```python
from build123d import *

# Parameters (mm, degrees)
BOSS_EXTRUDE1_DEPTH = 55
SKETCH2_W           = 14.545162339
SKETCH2_H           = 14.545162338
CUT_EXTRUDE1_DEPTH  = 55
SKETCH3_W           = 7.673243051
SKETCH3_H           = 2.777107306
SKETCH3_W_2         = 8.184792588
CUT_EXTRUDE2_DEPTH  = 55
SKETCH4_R           = 2.665972182
CUT_EXTRUDE3_DEPTH  = 20
FILLET1_R           = 12.5


with BuildPart() as part:
    # Sketch1 → Boss-Extrude1 (new body)
    with BuildSketch(Plane.XY):
        Polygon((41.400095641, 5), (28.900095641, 5), (-2.499905164, 5), (-2.499905164, 10), (-22.499903554, 10), (-22.499903554, 5), (-28.900095641, 5), (-41.400095641, 5), (-41.400095641, -10), (-28.900095641, -10), (28.900095641, -10), (41.400095641, -10), align=None)
    extrude(amount=BOSS_EXTRUDE1_DEPTH)

    # Sketch2 → Cut-Extrude1 (cut)
    with BuildSketch(Plane(origin=(0, 5, 0), x_dir=(1, 0, 0), z_dir=(0, 1, 0))):
        with Locations((23.65160359, -27.5)):
            Rectangle(SKETCH2_W, SKETCH2_H)
    extrude(amount=-CUT_EXTRUDE1_DEPTH, mode=Mode.SUBTRACT)

    # Sketch3 → Cut-Extrude2 (cut)
    with BuildSketch(Plane(origin=(-2.499905164, 0, 0), x_dir=(0, 0, -1), z_dir=(1, 0, 0))):
        with Locations((-47.272594324, 6.388553653)):
            Rectangle(SKETCH3_W, SKETCH3_H)
        with Locations((-8.522716918, 6.388553653)):
            Rectangle(SKETCH3_W_2, SKETCH3_H)
    extrude(amount=-CUT_EXTRUDE2_DEPTH, mode=Mode.SUBTRACT)

    # Sketch4 → Cut-Extrude3 (cut)
    with BuildSketch(Plane(origin=(41.400095641, 0, 0), x_dir=(0, 0, -1), z_dir=(1, 0, 0))):
        with Locations((-27.5, -2.516392759)):
            Circle(SKETCH4_R)
    extrude(amount=-CUT_EXTRUDE3_DEPTH, mode=Mode.SUBTRACT)

    # Fillet1
    fillet1_edges = [part.edges().sort_by_distance(p)[0] for p in [
        (-41.400095641, -2.5, 0),
        (41.400095641, -2.5, 0),
        (-41.400095641, -2.5, 55),
        (41.400095641, -2.5, 55),
    ]]
    fillet(fillet1_edges, radius=FILLET1_R)


solid = part.part
```
Work out the finished part from the listing and answer in its coordinate system (mm). A direction names the side the tool comes from. Give positions to 0.01 mm unless a question says otherwise; leave off trailing zeros. Order: outer loops, then holes, each group sorted by start corner. A loop starts at its lowest first (then second) coordinate and runs counter-clockwise, first axis right, second up. Notation, with made-up numbers: (62, 7.25) -> (81, 7.25) arc R23 cw to (81, 39.25) -> close; hole circle Ø10 at (-14.75, 79). An arc over 180 degrees is marked (long way). Answer as CSV lines item,"result". Start each with the question number.
(1) Consider line 1 along X through (y, z) = (-1, 21); line 2 along Y through (x, z) = (33.5, 27.5); line 3 along X through (y, z) = (8, 30). Determine where each line is inside the solid, lowest interval first.
(2) For a pull along X with two mould halves and no side action, classify faces 5 (the flat face through (-12, 7.777, 9)), 6 (the cylindrical face through (37.836, -2.395, 51.241)), 7 (the flat face through (-22.5, 8, 27)), 8 (the flat face through (24, -2, 20.227)) as released by +X, released by -X, zero draft, split by the parting line, or undercut.
(3) Section C-C, the plane x = -20.5 is taken. Write down the section's boundary in (y, z), plus the area to 3 significant figures.
(4) Section A-A, the plane z = 22.5 is taken. Write down the section's boundary in (x, y), plus the area to 3 significant figures.
(5) Each of these flat-tipped pins is pushed along its axis until it touches: pin 1 Ø1.5 at (y, z) = (6.5, 23.5) entering from -X; pin 2 Ø1.5 at (y, z) = (7.5, 14.5) entering from +X; pin 3 Ø1 at (x, z) = (0, 22) entering from +Y. Where does it stop, or does it pass through?
(6) Which of the six approach directions +Z, -Z, +X, -X, +Y, -Y give full straight-line access (tool end or side, diameter ignored) to faces 1 (the flat face through (24, -2, 34.773)), 2 (the cylindrical face through (36.235, -2.399, 30.163)), 3 (the flat face through (-12, 6, 43.436)), 4 (the flat face through (-1, -10, 27))?
(7) Section B-B, the plane x = 21.5 is taken. Write down the section's boundary in (y, z), plus the area to 3 significant figures.
(8) Section D-D, the plane y = 1.5 is taken. Write down the section's boundary in (x, z).
Entries:
1,line 1,"-41.4 to 16.38, 30.92 to 41.4"
1,line 2,"-10 to -5.18, 0.15 to 5"
1,line 3,"-22.5 to -2.5"
2,face 5,"zero draft"
2,face 6,"released by +X"
2,face 7,"released by -X"
2,face 8,"undercut"
3,outline,"(-10, 0) -> (10, 0) -> (10, 55) -> (-10, 55) -> close; hole (5, 4.43) -> (7.78, 4.43) -> (7.78, 12.62) -> (5, 12.62) -> close; hole (5, 43.44) -> (7.78, 43.44) -> (7.78, 51.11) -> (5, 51.11) -> close"
3,area,"1,060 mm²"
4,outline,"(-41.4, -10) -> (16.38, -10) -> (16.38, 5) -> (-2.5, 5) -> (-2.5, 10) -> (-22.5, 10) -> (-22.5, 5) -> (-41.4, 5) -> close; (30.92, -10) -> (41.4, -10) -> (41.4, 5) -> (30.92, 5) -> close"
4,area,"1,120 mm²"
5,pin 1,"x = -22.5"
5,pin 2,"x = -2.5"
5,pin 3,"y = 5"
6,face 1,"+Y, -Y"
6,face 2,"+X"
6,face 3,"+X, -X"
6,face 4,"+Z, -Z, +X, -X, -Y"
7,outline,"(-10, 0) -> (5, 0) -> (5, 20.23) -> (-10, 20.23) -> close; (-10, 34.77) -> (5, 34.77) -> (5, 55) -> (-10, 55) -> close"
7,area,"607 mm²"
8,outline,"(-41.4, 12.5) arc R12.5 ccw to (-28.9, 0) -> (28.9, 0) arc R12.5 ccw to (41.4, 12.5) -> (41.4, 42.5) arc R12.5 ccw to (28.9, 55) -> (-28.9, 55) arc R12.5 ccw to (-41.4, 42.5) -> close; hole (16.38, 20.23) -> (30.92, 20.23) -> (30.92, 34.77) -> (16.38, 34.77) -> close"
